Geometry: final body of the model. Coordinates: model frame, mm. A direction names the side the tool comes from. Round coordinates to 2 decimals unless told otherwise and drop trailing zeros. Loops run counter-clockwise (first coordinate to the right, second up) from the corner with the lowest first, then second, coordinate; pieces in that order, holes last. Notation, with made-up numbers: (28, 34) -> (56, 34) arc R17 cw to (56, 44) -> close; hole circle Ø8 at (-2, -5.5). An arc over 180 degrees is marked (long way). Answer in a Markdown table with one row per item.
```python
from build123d import *

# Parameters (mm, degrees)
F0_W     = 190.5
F0_H     = 101.6
F1_DEPTH = 3.175
F2_W     = 184.15
F2_H     = 3.175
F3_DEPTH = 53.975
F4_W     = 3.175
F4_H     = 95.25
F5_DEPTH = 53.975
F6_R     = 7.62
F7_R     = 7.62
F8_W     = 3.175
F8_H     = 95.25
F9_DEPTH = 53.975
F10_R    = 7.62
F11_R    = 7.62
F12_R    = 10.16


with BuildPart() as f1:
    # F0 (on Front) → F1 (new body)
    with BuildSketch(Plane.XZ):
        with Locations((13.3651066571, -10.7336564614)):
            Rectangle(F0_W, F0_H)
    extrude(amount=F1_DEPTH)

    # F2 (on face) → F3 (join)
    with BuildSketch(Plane.XZ.offset(3.175)):
        Polygon((108.6151066571, -61.5336564614), (108.6151066571, 40.0663435386), (105.4401066571, 40.0663435386), (105.4401066571, 36.8913435386), (105.4401066571, -58.3586564614), (105.4401066571, -61.5336564614), align=None)
        with Locations((13.3651066571, 38.4788435386)):
            Rectangle(F2_W, F2_H)
        Polygon((-78.7098933429, 36.8913435386), (-78.7098933429, 40.0663435386), (-81.8848933429, 40.0663435386), (-81.8848933429, -61.5336564614), (-78.7098933429, -61.5336564614), (-78.7098933429, -58.3586564614), align=None)
        with Locations((13.3651066571, -59.9461564614)):
            Rectangle(F2_W, F2_H)
    extrude(amount=F3_DEPTH)

    # F4 (on face) → F5 (join)
    with BuildSketch(Plane.XZ.offset(3.175)):
        with Locations((0.60594371, -10.7336564614)):
            Rectangle(F4_W, F4_H)
    extrude(amount=F5_DEPTH)

    # F6
    f6_edges = [f1.edges().sort_by_distance(p)[0] for p in [
        (-0.981556, -30.1625, -58.358656),
        (2.193444, -30.1625, 36.891344),
        (2.193444, -30.1625, -58.358656),
        (-0.981556, -30.1625, 36.891344),
    ]]
    fillet(f6_edges, radius=F6_R)

    # F7
    f7_edges = [f1.edges().sort_by_distance(p)[0] for p in [
        (-78.709893, -30.1625, -58.358656),
        (-78.709893, -30.1625, 36.891344),
    ]]
    fillet(f7_edges, radius=F7_R)

    # F8 (on face) → F9 (join)
    with BuildSketch(Plane.XZ.offset(3.175)):
        with Locations((26.2904159218, -10.7336564614)):
            Rectangle(F8_W, F8_H)
    extrude(amount=F9_DEPTH)

    # F10
    f10_edges = [f1.edges().sort_by_distance(p)[0] for p in [
        (24.702916, -30.1625, -58.358656),
        (24.702916, -30.1625, 36.891344),
        (27.877916, -30.1625, 36.891344),
        (27.877916, -30.1625, -58.358656),
    ]]
    fillet(f10_edges, radius=F10_R)

    # F11
    f11_edges = [f1.edges().sort_by_distance(p)[0] for p in [
        (105.440107, -30.1625, 36.891344),
        (105.440107, -30.1625, -58.358656),
    ]]
    fillet(f11_edges, radius=F11_R)

    # F12
    f12_edges = [f1.edges().sort_by_distance(p)[0] for p in [
        (-81.884893, -28.575, -61.533656),
        (108.615107, -28.575, -61.533656),
        (108.615107, -28.575, 40.066344),
        (-81.884893, -28.575, 40.066344),
    ]]
    fillet(f12_edges, radius=F12_R)


solid = f1.part
```
Item 1: Ray query, L1, parallel to X at y = -46.5, z = 8.5; L2, parallel to Z at x = 39, y = -24; L3, parallel to Y at x = -7, z = 19.5 (3 decimals). Return the intervals inside material, ascending.
Ans:
| item | result |
|---|---|
| L1 | -81.88 to -78.71, -0.98 to 2.19, 24.7 to 27.88, 105.44 to 108.62 |
| L2 | -61.53 to -58.36, 36.89 to 40.07 |
| L3 | -3.175 to 0 |
Item 2: Section query C-C, the plane z = 22.5. Output: boundary loops of the cut face in (x, y) (3 decimals).
Ans:
| item | result |
|---|---|
| outline | (-81.885, -57.15) -> (-78.71, -57.15) -> (-78.71, -3.175) -> (-0.982, -3.175) -> (-0.982, -57.15) -> (2.193, -57.15) -> (2.193, -3.175) -> (24.703, -3.175) -> (24.703, -57.15) -> (27.878, -57.15) -> (27.878, -3.175) -> (105.44, -3.175) -> (105.44, -57.15) -> (108.615, -57.15) -> (108.615, 0) -> (-81.885, 0) -> close |
Item 3: Set-up query: faces 4 (the flat face through (27.878, -30, -11)), 5 (the cylindrical face through (-78.988, -28.175, -58.478)). Return all of +Z, -Z, +X, -X, +Y, -Y with unobstructed straight access to the full face (end or side cutting, diameter ignored); none if empty.
Ans:
| item | result |
|---|---|
| face 4 | -Y |
| face 5 | -Z, -X, +Y, -Y |
Item 4: First-contact query: P1, Ø23.5, axis at x = -53, z = -1, coming from the -Y side (3 decimals). Flat tip, straight axial feed; report the tip coordinate or a pass-through.
Ans:
| item | result |
|---|---|
| P1 | y = -3.175 |
Item 5: Section query D-D, the plane z = -54.5. Output: boundary loops of the cut face in (x, y) (3 decimals), and give its area (3 significant figures).
Ans:
| item | result |
|---|---|
| outline | (-81.392, -57.15) -> (-77.717, -57.15) -> (-77.717, -3.175) -> (-1.975, -3.175) -> (-1.975, -57.15) -> (3.186, -57.15) -> (3.186, -3.175) -> (23.71, -3.175) -> (23.71, -57.15) -> (28.871, -57.15) -> (28.871, -3.175) -> (104.447, -3.175) -> (104.447, -57.15) -> (108.122, -57.15) -> (108.122, 0) -> (-81.392, 0) -> close |
| area | 1,560 mm2 |
Item 6: Section query B-B, the plane x = -67. Output: boundary loops of the cut face in (y, z) (3 decimals).
Ans:
| item | result |
|---|---|
| outline | (-57.15, -61.534) -> (0, -61.534) -> (0, 40.066) -> (-57.15, 40.066) -> (-57.15, 36.891) -> (-3.175, 36.891) -> (-3.175, -58.359) -> (-57.15, -58.359) -> close |
Item 7: Section query A-A, the plane y = -29. State how many separate pieces and enclosed holes the cut face has, and give its area (3 significant figures).
Ans:
| item | result |
|---|---|
| separate pieces | 1 |
| enclosed holes | 3 |
| area | 2,480 mm2 |
Item 8: Mould query, pull axis X, two halves, no side actions, for faces 1 (the flat face through (27, -57.15, -10)), 2 (the cylindrical face through (105.718, -28.175, -58.478)), 3 (the cylindrical face through (30.169, -30.54, -56.186)). Classes: released by +X, released by -X, zero draft, split by the parting line, or undercut.
Ans:
| item | result |
|---|---|
| face 1 | zero draft |
| face 2 | released by +X |
| face 3 | undercut |
